Input: part model. Units: mm. Frame: model coordinates. A direction names the side the tool comes from. Coordinates: 2 decimals unless noted, no trailing zeros. Loops run counter-clockwise (first coordinate to the right, second up) from the corner with the lowest first, then second, coordinate; pieces in that order, holes last. Notation, with made-up numbers: (62, -40) -> (74, -40) arc R23 cw to (74, -10) -> close; hole circle Ø4 at (-34.75, 2). An arc over 180 degrees is marked (long way). Put each result on its own line as item: value. Start each with the question number.
1) Cut plane B-B (x = 0). Return the cut outline in (y, z), plus the area to 3 significant figures.
2) Cut plane A-A (z = 0). Return the cut outline in (x, y), plus the area to 3 significant figures.
3) Material intervals for L1, parallel to Z at x = -16, y = 3.5; L2, parallel to Z at x = 14.5, y = 2.5; L3, parallel to X at y = 5.75, z = 0, sorted ascending.
4) Cut plane D-D (y = 5.75). Return the cut outline in (x, z), plus the area to 3 significant figures.
5) Pull-direction query (X, two-part tool) for faces 4 (the flat face through (9.4, 0, -9.4)), 5 (the cylindrical face through (-39.05, 3.7, -8.67)), 6 (the flat face through (-17, 8.5, 17)); classes: pulls with the +X half, pulls with the -X half, needs draft (parallel to the pull), parting line crosses it, or undercut.
6) Cut plane C-C (y = 10.5). Return the cut outline in (x, z), plus the area to 3 significant figures.
7) Contact query for flat-ended pins moving along their axis: P1, Ø3, axis at x = -10, y = 8, coming from the +Z side; P2, Ø11, axis at x = -15.56, z = -15.56, coming from the -Y side; P3, Ø6, axis at y = 6.5, z = 12.5, coming from the -X side; P4, Ø1, axis at y = 7, z = -10, coming from the +X side. Output: stop coordinate, or through.
8) Set-up query: faces 1 (the cylindrical face through (-7.91, 4.19, -10.316)), 2 (the flat face through (14, 8.5, 17)), 3 (the cylindrical face through (-9.76, 9.98, -2.17)). Return all of +Z, -Z, +X, -X, +Y, -Y with unobstructed straight access to the full face (end or side cutting, diameter ignored); none if empty.
from build123d import *

# Parameters (mm, degrees)
SKETCH1_R           = 40
SKETCH1_R_2         = 13
BOSS_EXTRUDE1_DEPTH = 8.5
SKETCH3_R           = 1.75
CUT_EXTRUDE1_DEPTH  = 58.203583804
SKETCH2_R           = 40
SKETCH2_R_2         = 10
SKETCH2_R_3         = 3.5
BOSS_EXTRUDE2_DEPTH = 3
FILLET1_R           = 4


with BuildPart() as part:
    # Sketch1 → Boss-Extrude1 (new body)
    with BuildSketch(Plane(origin=(0, 0, 0), x_dir=(1, 0, 0), z_dir=(0, 1, 0))):
        with Locations(Location((0, 0, 0), (0, 0, 270))):
            Circle(SKETCH1_R)
        with Locations(Location((0, 0, 0), (0, 0, 270))):
            Circle(SKETCH1_R_2, mode=Mode.SUBTRACT)
    extrude(amount=BOSS_EXTRUDE1_DEPTH)

    # Sketch3 → Cut-Extrude1 (cut, through all)
    with BuildSketch(Plane(origin=(0, 8.5, 0), x_dir=(1, 0, 0), z_dir=(0, 1, 0))):
        with Locations(Location((-15.556349186, 15.556349186, 0), (0, 0, 270))):
            Circle(SKETCH3_R)
        with Locations(Location((15.556349186, 15.556349186, 0), (0, 0, 270))):
            Circle(SKETCH3_R)
        with Locations(Location((15.556349186, -15.556349186, 0), (0, 0, 270))):
            Circle(SKETCH3_R)
        with Locations(Location((-15.556349186, -15.556349186, 0), (0, 0, 270))):
            Circle(SKETCH3_R)
    extrude(amount=-CUT_EXTRUDE1_DEPTH, mode=Mode.SUBTRACT)

    # Sketch2 → Boss-Extrude2 (add)
    with BuildSketch(Plane(origin=(0, 8.5, 0), x_dir=(1, 0, 0), z_dir=(0, 1, 0))):
        with Locations(Location((0, 0, 0), (0, 0, 270))):
            Circle(SKETCH2_R)
        with Locations(Location((0, 0, 0), (0, 0, 270))):
            Circle(SKETCH2_R_2, mode=Mode.SUBTRACT)
        with Locations(Location((-15.556349186, 15.556349186, 0), (0, 0, 270))):
            Circle(SKETCH2_R_3, mode=Mode.SUBTRACT)
        with Locations(Location((15.556349186, 15.556349186, 0), (0, 0, 270))):
            Circle(SKETCH2_R_3, mode=Mode.SUBTRACT)
        with Locations(Location((15.556349186, -15.556349186, 0), (0, 0, 270))):
            Circle(SKETCH2_R_3, mode=Mode.SUBTRACT)
        with Locations(Location((-15.556349186, -15.556349186, 0), (0, 0, 270))):
            Circle(SKETCH2_R_3, mode=Mode.SUBTRACT)
    extrude(amount=BOSS_EXTRUDE2_DEPTH)

    # Fillet1
    fillet1_edges = [part.edges().sort_by_distance(p)[0] for p in [
        (0, 11.5, -40),
    ]]
    fillet(fillet1_edges, radius=FILLET1_R)


solid = part.part
Results found:
1. outline: (0, -40) -> (7.5, -40) arc R4 ccw to (11.5, -36) -> (11.5, -10) -> (8.5, -10) -> (8.5, -13) -> (0, -13) -> close; (0, 13) -> (8.5, 13) -> (8.5, 10) -> (11.5, 10) -> (11.5, 36) arc R4 ccw to (7.5, 40) -> (0, 40) -> close
1. area: 632 mm2
2. outline: (-40, 0) -> (-13, 0) -> (-13, 8.5) -> (-10, 8.5) -> (-10, 11.5) -> (-36, 11.5) arc R4 ccw to (-40, 7.5) -> close; (10, 8.5) -> (13, 8.5) -> (13, 0) -> (40, 0) -> (40, 7.5) arc R4 ccw to (36, 11.5) -> (10, 11.5) -> close
2. area: 632 mm2
3. L1: z = -36.66 to -17.25, -13.86 to 13.86, 17.25 to 36.66
3. L2: z = -37.28 to -16.95, -14.16 to 14.16, 16.95 to 37.28
3. L3: x = -40 to -13, 13 to 40
4. outline: circle Ø80 at (0, 0); hole circle Ø3.5 at (-15.56, -15.56); hole circle Ø3.5 at (-15.56, 15.56); hole circle Ø26 at (0, 0); hole circle Ø3.5 at (15.56, -15.56); hole circle Ø3.5 at (15.56, 15.56)
4. area: 4,460 mm2
5. face 4: needs draft
5. face 5: parting line crosses it
5. face 6: undercut
6. outline: circle Ø77.29 at (0, 0); hole circle Ø7 at (-15.56, -15.56); hole circle Ø7 at (-15.56, 15.56); hole circle Ø20 at (0, 0); hole circle Ø7 at (15.56, -15.56); hole circle Ø7 at (15.56, 15.56)
6. area: 4,220 mm2
7. P1: stops at z = 39.07
7. P2: stops at y = 0
7. P3: stops at x = -38.86
7. P4: stops at x = 38.86
8. face 1: -Y
8. face 2: +Y
8. face 3: +Y, -Y
